Model file for the job. Use its own axes, mm. A direction names the side the tool comes from. Round coordinates to 2 decimals unless told otherwise and drop trailing zeros. Order: outer loops, then holes, each group sorted by start corner. A loop starts at its lowest first (then second) coordinate and runs counter-clockwise, first axis right, second up. Notation, with made-up numbers: (54, 49) -> (90, 49) arc R18 cw to (90, 82) -> close; hole circle Ø8 at (35.5, 72). An arc over 180 degrees is marked (long way). Use CSV: the item, a comma, the result in double quotes.
```python
from build123d import *

# Parameters (mm, degrees)
SKETCH1_R           = 50.8
BOSS_EXTRUDE1_DEPTH = 254
CUT_EXTRUDE1_START  = -86.25332
SKETCH2_R           = 19.05
CUT_EXTRUDE1_DEPTH  = 3.175
CUT_EXTRUDE2_START  = 83.07832
SKETCH4_R           = 19.05
CUT_EXTRUDE2_DEPTH  = 3.175


with BuildPart() as part:
    # Sketch1 → Boss-Extrude1 (new body)
    with BuildSketch(Plane.XY):
        Circle(SKETCH1_R)
    extrude(amount=BOSS_EXTRUDE1_DEPTH)

    # Sketch2 → Cut-Extrude1 (cut)
    with BuildSketch(Plane.XY.offset(254).offset(CUT_EXTRUDE1_START)):
        with BuildLine():
            ThreePointArc((-12.600390619, 49.2125), (-35.921024484, 35.921024484), (-49.2125, 12.600390619))
            ThreePointArc((-49.2125, 12.600390619), (-38.1, 0), (-49.2125, -12.600390619))
            ThreePointArc((-49.2125, -12.600390619), (-35.921024484, -35.921024484), (-12.600390619, -49.2125))
            ThreePointArc((-12.600390619, -49.2125), (0, -38.1), (12.600390619, -49.2125))
            ThreePointArc((12.600390619, -49.2125), (35.921024484, -35.921024484), (49.2125, -12.600390619))
            ThreePointArc((49.2125, -12.600390619), (38.1, 0), (49.2125, 12.600390619))
            ThreePointArc((49.2125, 12.600390619), (35.921024484, 35.921024484), (12.600390619, 49.2125))
            ThreePointArc((12.600390619, 49.2125), (0, 38.1), (-12.600390619, 49.2125))
        make_face()
        Circle(SKETCH2_R, mode=Mode.SUBTRACT)
    extrude(amount=CUT_EXTRUDE1_DEPTH, mode=Mode.SUBTRACT)

    # Sketch4 → Cut-Extrude2 (cut)
    with BuildSketch(Plane.XY.offset(CUT_EXTRUDE2_START)):
        with BuildLine():
            ThreePointArc((-12.600390619, 49.2125), (-35.921024484, 35.921024484), (-49.2125, 12.600390619))
            ThreePointArc((-49.2125, 12.600390619), (-38.1, 0), (-49.2125, -12.600390619))
            ThreePointArc((-49.2125, -12.600390619), (-35.921024484, -35.921024484), (-12.600390619, -49.2125))
            ThreePointArc((-12.600390619, -49.2125), (0, -38.1), (12.600390619, -49.2125))
            ThreePointArc((12.600390619, -49.2125), (35.921024484, -35.921024484), (49.2125, -12.600390619))
            ThreePointArc((49.2125, -12.600390619), (38.1, 0), (49.2125, 12.600390619))
            ThreePointArc((49.2125, 12.600390619), (35.921024484, 35.921024484), (12.600390619, 49.2125))
            ThreePointArc((12.600390619, 49.2125), (0, 38.1), (-12.600390619, 49.2125))
        make_face()
        Circle(SKETCH4_R, mode=Mode.SUBTRACT)
    extrude(amount=CUT_EXTRUDE2_DEPTH, mode=Mode.SUBTRACT)


solid = part.part
```
Q1. Probe line 1 along Z through (x, y) = (45.5, 12.5); line 2 along Y through (x, z) = (-2, 134.5). List the from-to ranges inside material, lowest first.
From the geometry:
line 1,"z = 0 to 83.08, 86.25 to 167.75, 170.92 to 254"
line 2,"y = -50.76 to 50.76"
Q2. Cut at B-B (y = 42). Give the cut face in (x, z).
From the geometry:
outline,"(-28.58, 0) -> (28.58, 0) -> (28.58, 83.08) -> (9.16, 83.08) -> (9.16, 86.25) -> (28.58, 86.25) -> (28.58, 167.75) -> (9.16, 167.75) -> (9.16, 170.92) -> (28.58, 170.92) -> (28.58, 254) -> (-28.58, 254) -> (-28.58, 170.92) -> (-9.16, 170.92) -> (-9.16, 167.75) -> (-28.58, 167.75) -> (-28.58, 86.25) -> (-9.16, 86.25) -> (-9.16, 83.08) -> (-28.58, 83.08) -> close"
Q3. Pin check, flat tips, straight feed: pin 1 (5 mm diameter, centred on y = -35, z = 190.5, fed in from -X); pin 2 (6 mm diameter, centred on y = -33, z = 70, fed in from +X); pin 3 (10 mm diameter, centred on x = -21.5, z = 27, fed in from -Y); pin 4 (4 mm diameter, centred on y = 0.5, z = 207.5, fed in from -X). Stop position of each tip, or through.
From the geometry:
pin 1,"stops at x = -39.04"
pin 2,"stops at x = 41"
pin 3,"stops at y = -48.05"
pin 4,"stops at x = -50.8"
Q4. Mould opens along X. For faces 3 (the cylindrical face through (-11.012, -49.592, 125.222)), 4 (the flat face through (21, 1, 167.747)), 5 (the flat face through (-1, 1, 254)) say: +X half, -X half, draft (parallel to the pull), parting line (faces both ways), or undercut.
From the geometry:
face 3,"parting line"
face 4,"undercut"
face 5,"draft"
Q5. Cut at C-C (z = 60). Give the cut face in (x, y).
From the geometry:
outline,"circle Ø101.6 at (0, 0)"
Q6. Which spindle directions (+Z, -Z, +X, -X, +Y, -Y) get a long thin tool onto all of the face, cutting with end or side? Do faces 1 (the flat face through (21, 1, 170.922)), 2 (the flat face through (-1, 1, 0)). Say none if no direction does.
From the geometry:
face 1,"none"
face 2,"-Z, +X, -X, +Y, -Y"
Q7. Cut at A-A (x = -9). Give the cut face in (y, z), plus the area to 3 significant figures.
From the geometry:
outline,"(-50, 0) -> (50, 0) -> (50, 254) -> (-50, 254) -> close; hole (-41.84, 83.08) -> (-16.79, 83.08) -> (-16.79, 86.25) -> (-41.84, 86.25) -> close; hole (-41.84, 167.75) -> (-16.79, 167.75) -> (-16.79, 170.92) -> (-41.84, 170.92) -> close; hole (16.79, 83.08) -> (41.84, 83.08) -> (41.84, 86.25) -> (16.79, 86.25) -> close; hole (16.79, 167.75) -> (41.84, 167.75) -> (41.84, 170.92) -> (16.79, 170.92) -> close"
area,"25,100 mm²"
Q8. Cut at D-D (x = 43). Give the cut face in (y, z).
From the geometry:
outline,"(-27.05, 0) -> (27.05, 0) -> (27.05, 83.08) -> (10.02, 83.08) -> (10.02, 86.25) -> (27.05, 86.25) -> (27.05, 167.75) -> (10.02, 167.75) -> (10.02, 170.92) -> (27.05, 170.92) -> (27.05, 254) -> (-27.05, 254) -> (-27.05, 170.92) -> (-10.02, 170.92) -> (-10.02, 167.75) -> (-27.05, 167.75) -> (-27.05, 86.25) -> (-10.02, 86.25) -> (-10.02, 83.08) -> (-27.05, 83.08) -> close"
